```python
from build123d import *

# Parameters (mm, degrees)
SKETCH_1_W          = 73
SKETCH_1_H          = 90
EXTRUDE_1_DEPTH     = 4
MM_1_D              = 3
MM_1_CSINK_D        = 3.05
MM_1_CSINK_ANGLE    = 100
SKETCH_5_R          = 17.5
CUT_EXTRUDE_3_DEPTH = 116.952576513
SKETCH_9_R          = 23.5
CUT_EXTRUDE_4_DEPTH = 2
SKETCH_10_W         = 19
SKETCH_10_H         = 6
CUT_EXTRUDE_5_DEPTH = 10
FILLET_1_R          = 1


with BuildPart() as part:
    # 草图1 → 凸台-拉伸1 (new body)
    with BuildSketch(Plane.XY):
        with Locations((36.5, 45)):
            Rectangle(SKETCH_1_W, SKETCH_1_H)
    extrude(amount=EXTRUDE_1_DEPTH)

    # 大小mm 暗销孔1 (through all)
    with Locations(Plane.XY.offset(4)):
        with Locations((2.5, 2.5), (70.5, 2.5), (70.5, 87.5), (2.5, 87.5)):
            CounterSinkHole(MM_1_D / 2, MM_1_CSINK_D / 2, counter_sink_angle=MM_1_CSINK_ANGLE)

    # 草图5 → 切除-拉伸3 (cut, through all)
    with BuildSketch(Plane.XY.offset(4)):
        with Locations((36.5, 55)):
            Circle(SKETCH_5_R)
    extrude(amount=-CUT_EXTRUDE_3_DEPTH, mode=Mode.SUBTRACT)

    # 草图9 → 切除-拉伸4 (cut)
    with BuildSketch(Plane.XY.offset(4)):
        with Locations((36.5, 55)):
            Circle(SKETCH_9_R)
    extrude(amount=-CUT_EXTRUDE_4_DEPTH, mode=Mode.SUBTRACT)

    # 草图10 → 切除-拉伸5 (cut)
    with BuildSketch(Plane.XY.offset(4)):
        with Locations((36.5, 13)):
            Rectangle(SKETCH_10_W, SKETCH_10_H)
    extrude(amount=-CUT_EXTRUDE_5_DEPTH, mode=Mode.SUBTRACT)

    # 圆角1
    fillet_1_edges = [part.edges().sort_by_distance(p)[0] for p in [
        (73, 45, 4),
        (36.5, 90, 4),
        (0, 45, 4),
        (13, 55, 4),
        (19, 55, 2),
        (36.5, 10, 0),
        (46, 13, 0),
        (36.5, 16, 0),
        (27, 13, 0),
        (27, 13, 4),
        (36.5, 10, 4),
        (46, 13, 4),
        (36.5, 16, 4),
        (36.5, 0, 4),
    ]]
    fillet(fillet_1_edges, radius=FILLET_1_R)


solid = part.part
```
Can you work these out from the model? Positions are in its coordinate system, mm. A direction names the side the tool comes from. Coordinates: 2 decimals unless noted, no trailing zeros. Loops run counter-clockwise (first coordinate to the right, second up) from the corner with the lowest first, then second, coordinate; pieces in that order, holes last. Notation, with made-up numbers: M -15,-11.5 L 1,-11.5 A20 ccw 1,16.5 Z; hole C 59.5,52.25 d1. An arc over 180 degrees is marked long. Put each result on its own line as item: value. Start each with the question number.
(1) Imagine slicing it at C-C on y = 55. List the corners of the cut face in (x, z) for me, and give its area (3 significant figures).
(2) We'd pull the mould along X, two halves only. Please class faces 1 (the face through (1.81, 1.17, 1.96)), 2 (the face through (33.44, 78.3, 2.51)), 3 (the face through (73, 44, 1)), 4 (the face through (0, 44, 1)): +X half, -X half, draft (parallel to the pull), parting line (faces both ways), or undercut.
(3) Which directions (+Z, -Z, +X, -X, +Y, -Y) give clear straight access to the entire face, cutting with the end or side of a thin tool? Please do faces 5 (the face through (47, 39, 2)), 6 (the face through (36, 0, 1)), 7 (the face through (46, 13, 2)).
(4) Imagine slicing it at A-A on x = 36.5. List the corners of the cut face in (y, z) for me.
(5) Will these pins go through, and if not, where does the flat tip stop? pin 1 Ø1.8 at (x, y) = (70.5, 87.5) entering from -Z; pin 2 Ø23.5 at (x, y) = (40, 65) entering from +Z.
(6) I need wall thicknesses on probe 1 along Y at (x, z) = (70.5, 1.3); probe 2 along X at (y, z) = (2.5, 2.95); probe 3 along Y at (x, z) = (36.5, 0.4). Which ranges of each line are inside material? Lowest first, please.
(7) Imagine slicing it at B-B on y = 13. List the corners of the cut face in (x, z) for me, and give its area (3 significant figures).
Worked answers:
1. outline: M 0,0 L 19,0 L 19,1 A1 ccw 18,2 L 13,2 L 13,3 A1 ccw 12,4 L 1,4 A1 ccw 0,3 Z; M 54,0 L 73,0 L 73,3 A1 ccw 72,4 L 61,4 A1 ccw 60,3 L 60,2 L 55,2 A1 ccw 54,1 Z
1. area: 127 mm2
2. face 1: undercut
2. face 2: undercut
2. face 3: +X half
2. face 4: -X half
3. face 5: +Z
3. face 6: +Z, -Z, +X, -X, -Y
3. face 7: +Z, -Z
4. outline: M 0,0 L 9,0 A1 ccw 10,1 L 10,3 A1 ccw 9,4 L 1,4 A1 ccw 0,3 Z; M 16,1 A1 ccw 17,0 L 37.5,0 L 37.5,1 A1 ccw 36.5,2 L 31.5,2 L 31.5,3 A1 ccw 30.5,4 L 17,4 A1 ccw 16,3 Z; M 72.5,0 L 90,0 L 90,3 A1 ccw 89,4 L 79.5,4 A1 ccw 78.5,3 L 78.5,2 L 73.5,2 A1 ccw 72.5,1 Z
5. pin 1: passes through
5. pin 2: stops at z = 2
6. probe 1: y = 0 to 1, 4 to 86, 89 to 90
6. probe 2: x = 0 to 1, 4 to 69, 72 to 73
6. probe 3: y = 0 to 9.8, 16.2 to 37.5, 72.5 to 90
7. outline: M 0,0 L 26,0 A1 ccw 27,1 L 27,3 A1 ccw 26,4 L 1,4 A1 ccw 0,3 Z; M 46,1 A1 ccw 47,0 L 73,0 L 73,3 A1 ccw 72,4 L 47,4 A1 ccw 46,3 Z
7. area: 215 mm2
